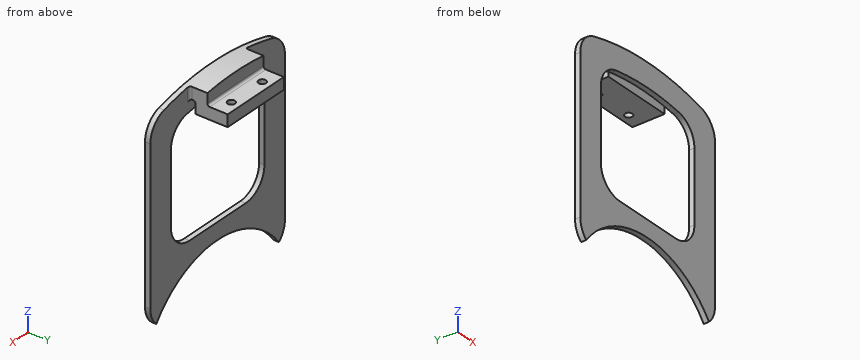
```python
from build123d import *

# Parameters (mm, degrees)
EXTRUDE_1_DEPTH             = 2.2000000000000006
EXTRUDE_2_DEPTH             = 16.000000000000004
SKETCH_3_W                  = 30
SKETCH_3_H                  = 13.500000000000002
EXTRUDE_3_DEPTH             = 5
CUT_EXTRUDE_START           = -8.5
CUT_EXTRUDE_1_DEPTH         = 8.5
CUT_EXTRUDE_2_DEPTH         = 88.46305189948819
HOLE_WIZARD_3_1_3_1_1_D     = 3.1
HOLE_WIZARD_3_1_3_1_1_DEPTH = 11.041658668
FILLET_1_R                  = 1
FILLET_2_R                  = 10


with BuildPart() as part:
    # 草图1 → 凸台-拉伸1 (new body)
    with BuildSketch(Plane.XZ.offset(11.45)):
        with BuildLine():
            Line((-27.748687791341045, 4.896974351176933), (-27.748687791341048, -66.4009079535447))
            ThreePointArc((-27.748687791341048, -66.4009079535447), (-26.915275099995267, -70.3976162382234), (-24.55395236877715, -73.7281430412905))
            ThreePointArc((-24.55395236877715, -73.7281430412905), (8.250000000000021, -56.98000000000004), (41.0539523687772, -73.7281430412905))
            ThreePointArc((41.0539523687772, -73.7281430412905), (43.41527509999529, -70.3976162382234), (44.24868779134105, -66.4009079535447))
            Line((44.24868779134105, -66.4009079535447), (44.24868779134099, 4.896974351176947))
            ThreePointArc((44.24868779134099, 4.896974351176947), (8.249999999999982, 11.041658667751605), (-27.748687791341045, 4.896974351176933))
        make_face()
    extrude(amount=-EXTRUDE_1_DEPTH)

    # 草图2 → 凸台-拉伸2 (add)
    with BuildSketch(Plane(origin=(0, -9.25, 0), x_dir=(-1, 0, 0), z_dir=(0, 1, 0))):
        with BuildLine():
            Line((6.75, 5), (-23.25, 5))
            Line((-23.25, 5), (-23.25, 9.99999999999994))
            ThreePointArc((-23.25, 9.99999999999994), (-8.249999999999993, 11.041658667751605), (6.749999999999999, 9.99999999999994))
            Line((6.749999999999999, 9.99999999999994), (6.75, 5))
        make_face()
    extrude(amount=EXTRUDE_2_DEPTH)

    # 草图3 → 凸台-拉伸3 (add)
    with BuildSketch(Plane(origin=(0, 0, 5), x_dir=(-1, 0, 0), z_dir=(0, 0, -1))):
        with Locations((-8.25, 0)):
            Rectangle(SKETCH_3_W, SKETCH_3_H)
    extrude(amount=EXTRUDE_3_DEPTH)

    # 草图4 → 切除-拉伸1 (cut)
    with BuildSketch(Plane(origin=(0, 6.750000000000004, 0), x_dir=(-1, 0, 0), z_dir=(0, 1, 0)).offset(CUT_EXTRUDE_START)):
        with BuildLine():
            Line((-23.25, 9.99999999999994), (-23.25, 5))
            Line((-23.25, 5), (6.75, 5))
            Line((6.75, 5), (6.749999999999999, 9.99999999999994))
            ThreePointArc((6.749999999999999, 9.99999999999994), (-8.249999999999993, 11.041658667751605), (-23.25, 9.99999999999994))
        make_face()
    extrude(amount=CUT_EXTRUDE_1_DEPTH, mode=Mode.SUBTRACT)

    # 草图5 → 切除-拉伸2 (cut, through all)
    with BuildSketch(Plane(origin=(0, -9.25, 0), x_dir=(-1, 0, 0), z_dir=(0, 1, 0))):
        with BuildLine():
            Line((-33.25000000000001, -2.0737612102855603), (-33.25, -50))
            Line((-33.25, -50), (16.75, -50))
            Line((16.75, -50), (16.749999999999993, -2.073761210285574))
            ThreePointArc((16.749999999999993, -2.073761210285574), (-8.249999999999995, 1.1473308976777048), (-33.25000000000001, -2.0737612102855603))
        make_face()
    extrude(amount=-CUT_EXTRUDE_2_DEPTH, mode=Mode.SUBTRACT)

    # Ø3.1 (3.1) 直径孔1
    with Locations(Plane(origin=(0, 0, 0), x_dir=(-1, 0, 0), z_dir=(0, 0, -1))):
        with Locations((-16.5, 3), (0, 3)):
            Hole(HOLE_WIZARD_3_1_3_1_1_D / 2, depth=HOLE_WIZARD_3_1_3_1_1_DEPTH)

    # 圆角1
    fillet_1_edges = [part.edges().sort_by_distance(p)[0] for p in [
        (-6.75, -9.25, 7.49999999999997),
        (23.25, -9.25, 7.49999999999997),
        (8.25, -9.25, 5),
        (8.25, -6.75, 5),
        (8.25, -1.7499999999999956, 5),
    ]]
    fillet(fillet_1_edges, radius=FILLET_1_R)

    # 圆角2
    fillet_2_edges = [part.edges().sort_by_distance(p)[0] for p in [
        (44.24868779134099, -10.35, 4.896974351176949),
        (-27.748687791341048, -10.35, 4.896974351176935),
        (33.25, -10.35, -2.0737612102855643),
        (-16.749999999999993, -10.35, -2.073761210285571),
        (-16.75, -10.35, -50),
        (33.25, -10.35, -50),
    ]]
    fillet(fillet_2_edges, radius=FILLET_2_R)


solid = part.part
```
The listing builds one solid part. Answer for the finished solid, in the listing's coordinates (mm). Coordinates: 2 decimals unless noted, no trailing zeros. Write each loop counter-clockwise with the first axis right and the second up, starting at its lowest first coordinate (ties: lowest second). Pieces come first, ordered by that corner, then holes. Notation, with made-up numbers: M -29,55 L 23,55 A20 ccw 23,88 Z; hole C 42,88 d6. An arc over 180 degrees is marked long. Use a Markdown table: item, result. Add a question column.
1. Section C-C (x = 0.5) is taken. Give the vertices of the cut face in (y, z), plus the area to 3 significant figures.
2. Given P1, Ø4, axis at x = 1.5, y = -1, coming from the -Z side; P2, Ø2.5, axis at x = 14, z = 9, coming from the +Y side; P3, Ø5, axis at y = -4, z = 3.5, coming from the -X side; P4, Ø12, axis at x = -8.5, z = -45.5, coming from the -Y side, each flat-ended and moving along its own axis, determine where each tip first touches the part or whether it passes through.
3. Section B-B (z = -42) is taken. Give the vertices of the cut face in (x, y), plus the area to 3 significant figures.
4. Section D-D (x = 12.5) is taken. Give the vertices of the cut face in (y, z), plus the area to 3 significant figures.
5. Section A-A (y = 3) is taken. Give the vertices of the cut face in (x, z).
6. Straight lines are drawn through the part: line 1 along Y through (x, z) = (16.5, 3.5); line 2 along X through (y, z) = (-5.75, 3); line 3 along Z through (x, y) = (3, 0.5). For each, find the intervals that lie inside material, in ascending order. Write a range as [from, to].
Data:
| question | item | result |
|---|---|---|
| 1 | outline | M -11.45,-57.73 L -9.25,-57.73 L -9.25,-50 L -11.45,-50 Z; M -11.45,0.84 L -9.25,0.84 L -9.25,4 A1 cw -8.25,5 L -7.75,5 A1 cw -6.75,4 L -6.75,0 L 1.53,0 L 1.53,5 L -0.75,5 A1 cw -1.75,6 L -1.75,10.76 L -11.45,10.76 Z; M 4.47,0 L 6.75,0 L 6.75,5 L 4.47,5 Z |
| 1 | area | 136 mm2 |
| 2 | P1 | stops at z = 0 |
| 2 | P2 | stops at y = -1.75 |
| 2 | P3 | stops at x = -6.75 |
| 2 | P4 | stops at y = -11.45 |
| 3 | outline | M -27.75,-11.45 L -16.55,-11.45 L -16.55,-9.25 L -27.75,-9.25 Z; M 33.05,-11.45 L 44.25,-11.45 L 44.25,-9.25 L 33.05,-9.25 Z |
| 3 | area | 49.3 mm2 |
| 4 | outline | M -11.45,-57.2 L -9.25,-57.2 L -9.25,-50 L -11.45,-50 Z; M -11.45,1.06 L -9.25,1.06 L -9.25,4 A1 cw -8.25,5 L -7.75,5 A1 cw -6.75,4 L -6.75,0 L 6.75,0 L 6.75,5 L -0.75,5 A1 cw -1.75,6 L -1.75,10.96 L -11.45,10.96 Z |
| 4 | area | 150 mm2 |
| 5 | outline | M -6.75,0 L -1.55,0 L -1.55,5 L -6.75,5 Z; M 1.55,0 L 14.95,0 L 14.95,5 L 1.55,5 Z; M 18.05,0 L 23.25,0 L 23.25,5 L 18.05,5 Z |
| 6 | line 1 | y = [-11.45, -9.25], [-6.75, 1.45], [4.55, 6.75] |
| 6 | line 2 | x = [-6.75, 23.25] |
| 6 | line 3 | z = [0, 5] |
